Autodesk Inventor part; units mm, degrees
ref_plane "YZ Plane" through (0, 0, 0) normal (1, 0, 0) x (0, 1, 0)
ref_plane "XZ Plane" through (0, 0, 0) normal (0, 1, 0) x (-1, 0, 0)
ref_plane "XY Plane" through (0, 0, 0) normal (0, 0, 1) x (1, 0, 0)
sketch "スケッチ1" plane through (0, 0, 0) normal (0, 0, 1) x (1, 0, 0)
  circle A0 centre (0, 0) radius 7
  circle A1 centre (-2.8284, 2.8284) radius 1.25
  circle A2 centre (-1.0353, -3.8637) radius 1.25
  circle A3 centre (3.8637, 1.0353) radius 1.25
  circle A4 centre (0, 0) radius 10
  line L0 (3.8637, 1.0353) -> (8.2104, 2.2) construction
  line L1 (4.2519, -0.4136) -> (8.5986, 0.7511)
  line L2 (7.8221, 3.6489) -> (3.4755, 2.4842)
  arc A5 (3.4755, 2.4842) -> (4.2519, -0.4136) centre (3.8637, 1.0353) ccw
  arc A6 (8.5986, 0.7511) -> (7.8221, 3.6489) centre (8.2104, 2.2) ccw
  line L3 (3.8637, 1.0353) -> (0, 0)
  line L4 (-7.0711, 4.9497) -> (-3.8891, 1.7678)
  arc A7 (-4.9497, 7.0711) -> (-7.0711, 4.9497) centre (-6.0104, 6.0104) ccw
  line L5 (-1.7678, 3.8891) -> (-4.9497, 7.0711)
  line L6 (-0.7511, -8.5986) -> (0.4136, -4.2519)
  arc A8 (-3.6489, -7.8221) -> (-0.7511, -8.5986) centre (-2.2, -8.2104) ccw
  line L7 (-2.4842, -3.4755) -> (-3.6489, -7.8221)
  point P0 (6.037, 1.6176)
  point P1 (6.2162, 3.2185)
  point P2 (6.9926, 0.3208)
  point P3 (-3.7741, 5.8954)
  point P4 (-5.8954, 3.7741)
  point P5 (-3.2185, -6.2162)
  point P6 (-0.3208, -6.9926)
  dimension "d0" = 14
  dimension "d1" = 2.5
  dimension "d2" = 4
  dimension "d5" = 360
  dimension "d9" = 20
  dimension "d18" = 3
  dimension "d21" = 360
extrude "押し出し1" add sketch "スケッチ1" along normal blind 5 contours A0 L2 A5 L1 | L1 A5 L2 A0
extrude "押し出し2" add sketch "スケッチ1" along normal blind 1.5 contours A0 L2 A6 L1 | L6 A8 L7 A0 | A0 L4 A7 L5
thread "ねじ1"
thread "ねじ2"
thread "ねじ3"
properties part number "アームカムAL" material "アルミニウム 2014-T4"
Can you work these out from the model? Positions are in its coordinate system, mm. A direction names the side the tool comes from. Round coordinates to 2 decimals unless told otherwise and drop trailing zeros. Write each loop counter-clockwise with the first axis right and the second up, starting at its lowest first coordinate (ties: lowest second). Pieces come first, ordered by that corner, then holes. Notation, with made-up numbers: M 21,-35.5 L 55,-35.5 A21 ccw 55,-20.5 Z; hole C -6,68 d10. An arc over 180 degrees is marked long. Use CSV: the item, a comma, the result in double quotes.
(1) Imagine slicing it at D-D (x = 6.5). Write out the boundary of the cut face in (y, z).
Check values:
outline,"M -2.6,0 L 3.29,0 L 3.29,1.5 L 2.6,1.5 L 2.6,5 L -2.6,5 Z"
(2) I need wall thicknesses on line 1 along X through (y, z) = (1, 0.35); line 2 along X through (y, z) = (0, 3.3); line 3 along Y through (x, z) = (-1, 2.5). Which ranges of each line are inside material? Lowest first, please.
Check values:
line 1,"-6.93 to 2.61, 5.11 to 9.11"
line 2,"-7 to 3.16, 4.56 to 7"
line 3,"-6.93 to -5.11, -2.61 to 6.93"
(3) We'd pull the mould along X, two halves only. Please class faces 5 (the flat face through (7.78, 0.53, 0.74)), 6 (the flat face through (-4.354, 6.475, 0.74)), 7 (the cylindrical face through (-3.82, 3.59, 2.46)), 8 (the flat face through (0, 0, 5)): +X half, -X half, draft (parallel to the pull), parting line (faces both ways), or undercut.
Check values:
face 5,"+X half"
face 6,"undercut"
face 7,"undercut"
face 8,"draft"
(4) Imagine slicing it at C-C (y = 2). Write out the boundary of the cut face in (x, z), plus the area to 3 significant figures.
Check values:
outline,"M -6.71,0 L -3.76,0 L -3.76,5 L -6.71,5 Z; M -1.89,0 L 3.07,0 L 3.07,5 L -1.89,5 Z; M 4.66,0 L 9.7,0 L 9.7,1.5 L 6.71,1.5 L 6.71,5 L 4.66,5 Z"
area,"54.3 mm^2"
(5) On a 3-axis mill with a long thin cutter (end or side, diameter ignored), from which of +Z, -Z, +X, -X, +Y, -Y can I reach the whole of each face in a straight line? I mean faces 1 (the flat face through (-6.49, 4.37, 0.74)), 2 (the flat face through (7.03, 3.437, 0.74)), 3 (the cylindrical face through (6.677, -2.103, 2.465)), 4 (the flat face through (-6, 6, 1.5)). Say none if no direction works.
Check values:
face 1,"+Z, -Z, -X"
face 2,"+Z, -Z, +Y"
face 3,"+Z"
face 4,"+Z, -X, +Y"
(6) Imagine slicing it at B-B (x = 0). Write out the boundary of the cut face in (y, z), plus the area to 3 significant figures.
Check values:
outline,"M -7,0 L -4.56,0 L -4.56,5 L -7,5 Z; M -3.16,0 L 7,0 L 7,5 L -3.16,5 Z"
area,"63.0 mm^2"
(7) I'm going to push flat-ended pins straight in: pin 1 (2 mm diameter, centred on y = -2, z = 3.5, fed in from -X); pin 2 (1 mm diameter, centred on x = 7.5, y = 1.5, fed in from +Z); pin 3 (1.5 mm diameter, centred on x = 4.5, z = 4.5, fed in from +Y). Where does each tip first touch, or does it pass through?
Check values:
pin 1,"x = -6.93"
pin 2,"z = 1.5"
pin 3,"y = 5.91"
(8) Imagine slicing it at A-A (y = 0). Write out the boundary of the cut face in (x, z).
Check values:
outline,"M -7,0 L 3.16,0 L 3.16,5 L -7,5 Z; M 4.56,0 L 7,0 L 7,5 L 4.56,5 Z"
